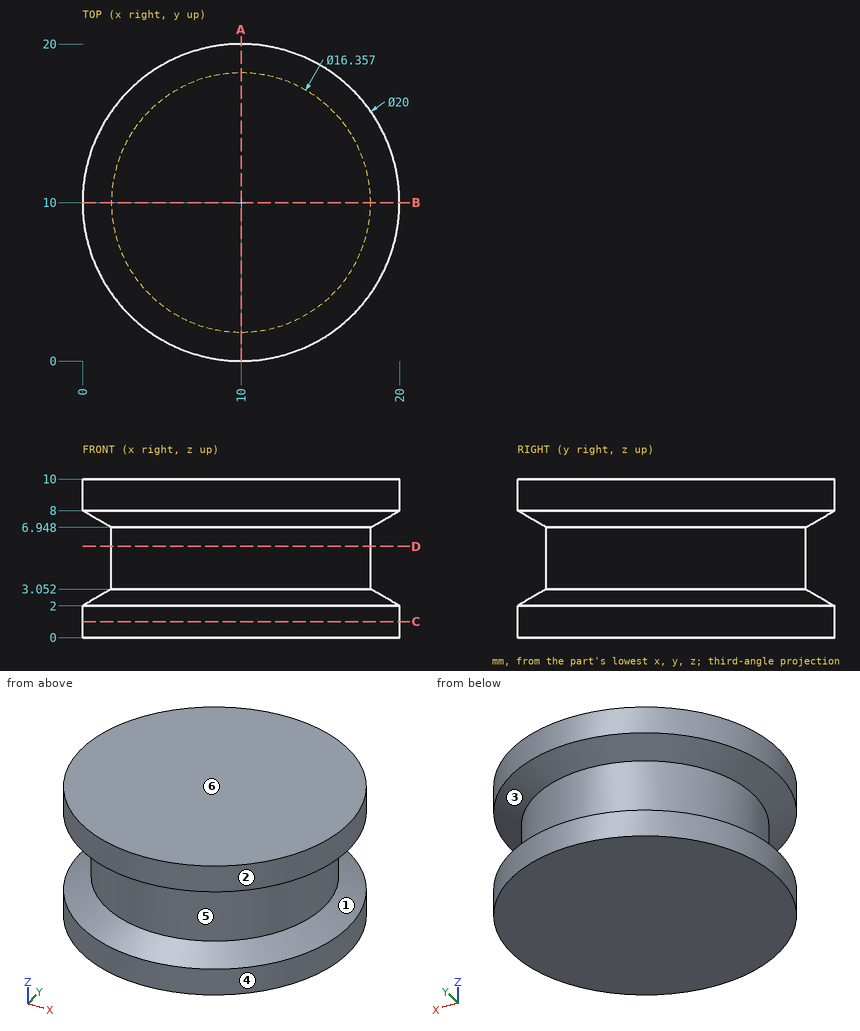
Geometry check sheet. Reference: drawing and pictorial views, mm from the part's lowest x, y, z. A direction names the side the tool comes from. Coordinates: 2 decimals unless noted, no trailing zeros. Loops run counter-clockwise (first coordinate to the right, second up) from the corner with the lowest first, then second, coordinate; pieces in that order, holes last. Notation, with made-up numbers: M -24,-35 L -12,-35 A29 ccw -12,-12 Z; hole C 41.5,-10.75 d1. An arc over 180 degrees is marked long. One line per item, written item: value.
1. Gauge pin test, flat ends, axial feed: P1, Ø5, axis at x = 8, z = 4, coming from the -Y side; P2, Ø6, axis at y = 13.5, z = 7, coming from the -X side; P3, Ø1, axis at x = 7, y = 11.5, coming from the -Z side; P4, Ø1, axis at x = 15.5, z = 3, coming from the +Y side (1 decimal). Record the tip position at first contact, or that the pin passes through.
Answers follow:
P1: y = 0.01
P2: x = 0.02
P3: z = 0
P4: y = 17.4
2. Material ranges on line 1 along Z through (x, y) = (2, 13.5); line 2 along Y through (x, z) = (14.75, 0.5); line 3 along Y through (x, z) = (10.25, 7.25) (1 decimal), recorded low to high. Write a range as from..to.
Answers follow:
line 1: 0..2.73, 7.27..10
line 2: 1.2..18.8
line 3: 1.3..18.7
3. Section check C-C on z = 1. Record the cut outline in (x, y), plus the area to 3 significant figures.
Answers follow:
outline: C 10,10 d20
area: 314 mm^2
4. Section check D-D on z = 5.75. Record the cut outline in (x, y), plus the area to 3 significant figures.
Answers follow:
outline: C 10,10 d16.36
area: 210 mm^2
5. Section check A-A on x = 10. Record the cut outline in (y, z), plus the area to 3 significant figures.
Answers follow:
outline: M 0,0 L 20,0 L 20,2 L 18.18,3.05 L 18.18,6.95 L 20,8 L 20,10 L 0,10 L 0,8 L 1.82,6.95 L 1.82,3.05 L 0,2 Z
area: 182 mm^2
6. Mould release check, pull along Z, two halves, no side actions. Record for the marked faces 3, 4, 5 and 6: pulls with the +Z half, pulls with the -Z half, needs draft (parallel to the pull), parting line crosses it, or undercut.
Answers follow:
face 3: undercut
face 4: needs draft
face 5: undercut
face 6: pulls with the +Z half
7. Set-up check for the marked faces 1 and 2: record each of +Z, -Z, +X, -X, +Y, -Y from which the full face is reachable in a straight line by a thin tool's end or side.
Answers follow:
face 1: none
face 2: +Z, -Z
